from build123d import *

# Parameters (mm, degrees)
F1_DEPTH = 10.5
F3_DEPTH = 2.25
F4_R     = 1


with BuildPart() as f1:
    # F0 (on Top) → F1 (new body)
    with BuildSketch(Plane.XY):
        with BuildLine():
            Line((16, 19), (-16, 19))
            ThreePointArc((-16, 19), (-21.6568542495, 16.6568542495), (-24, 11))
            Line((-24, 11), (-24, -11))
            ThreePointArc((-24, -11), (-21.6568542495, -16.6568542495), (-16, -19))
            Line((-16, -19), (16, -19))
            ThreePointArc((16, -19), (21.6568542495, -16.6568542495), (24, -11))
            Line((24, -11), (24, 11))
            ThreePointArc((24, 11), (21.6568542495, 16.6568542495), (16, 19))
        make_face()
    extrude(amount=F1_DEPTH)

    # F2 (on face) → F3 (join)
    with BuildSketch(Plane.XY.offset(10.5)):
        with BuildLine():
            Line((10, 21.85), (-16, 21.85))
            ThreePointArc((-16, 21.85), (-21.6568542495, 19.5068542495), (-24, 13.85))
            Line((-24, 13.85), (-24, 11))
            ThreePointArc((-24, 11), (-21.6568542495, 16.6568542495), (-16, 19))
            Line((-16, 19), (10, 19))
            Line((10, 19), (10, 21.85))
        make_face()
        with BuildLine():
            Line((10, -21.85), (10, -19))
            Line((10, -19), (-16, -19))
            ThreePointArc((-16, -19), (-21.6568542495, -16.6568542495), (-24, -11))
            Line((-24, -11), (-24, -13.85))
            ThreePointArc((-24, -13.85), (-21.6568542495, -19.5068542495), (-16, -21.85))
            Line((-16, -21.85), (10, -21.85))
        make_face()
    extrude(amount=-F3_DEPTH)

    # F4
    f4_edges = [f1.edges().sort_by_distance(p)[0] for p in [
        (10, -19, 9.375),
        (10, -21.85, 9.375),
        (10, 21.85, 9.375),
        (10, 19, 9.375),
    ]]
    fillet(f4_edges, radius=F4_R)


solid = f1.part
Design review of the part built by this model. Coordinates are the model's own, in mm. A direction names the side the tool comes from. Round coordinates to 2 decimals unless told otherwise and drop trailing zeros. Loops run counter-clockwise (first coordinate to the right, second up) from the corner with the lowest first, then second, coordinate; pieces in that order, holes last. Notation, with made-up numbers: (22, 68) -> (78, 68) arc R27 cw to (78, 104) -> close; hole circle Ø11 at (63.5, -20). An arc over 180 degrees is marked (long way). Use one line per item in the form item = value. Start each with the question number.
Q1. Machinability: for faces 1 (the face through (21.594, -16.719, 5.176)), 2 (the face through (-7, -20, 8.25)), 3 (the face through (-21.594, 16.719, 4.067)), which of the approach directions +Z, -Z, +X, -X, +Y, -Y give a long, thin tool a straight path to every point of the face, cutting with its end or side? Answer none if there is none.
Q2. Wall thickness on line 1 along Y through (x, z) = (-8, 3.75); line 2 along X through (y, z) = (12, 3.25); line 3 along X through (y, z) = (16, 4) (3 decimals): over which ranges is each line inside the solid? List them lowest first. Write a range as [from, to].
Q3. We need section A-A on z = 1. Give the boundary of the cut face in (x, y), then the cut area to 3 significant figures.
Q4. We need section B-B on x = -19. Give the boundary of the cut face in (y, z).
Q5. We need section D-D on x = 18. Give the boundary of the cut face in (y, z).
Q6. For pin 1 Ø1.5 at (x, y) = (14, 6.5) entering from -Z; pin 2 Ø3 at (y, z) = (-16, 5.5) entering from +X; pin 3 Ø5 at (x, z) = (-7.5, 3.5) entering from -Y; pin 4 Ø0.7 at (y, z) = (20.5, 9) entering from +X, all flat-tipped, find the tip position at first contact; note any pin that passes through.
Q7. We need section C-C on y = -16. Give the boundary of the cut face in (x, z) (3 decimals).
Calculated:
q1.face_1 = +Z, -Z, +X, -Y
q1.face_2 = -Z, -X, -Y
q1.face_3 = -Z, -X, +Y
q2.line_1 = [-19, 19]
q2.line_2 = [-23.94, 23.94]
q2.line_3 = [-22.245, 22.245]
q3.outline = (-24, -11) arc R8 ccw to (-16, -19) -> (16, -19) arc R8 ccw to (24, -11) -> (24, 11) arc R8 ccw to (16, 19) -> (-16, 19) arc R8 ccw to (-24, 11) -> close
q3.area = 1,770 mm²
q4.outline = (-21.27, 8.25) -> (-18.42, 8.25) -> (-18.42, 0) -> (18.42, 0) -> (18.42, 8.25) -> (21.27, 8.25) -> (21.27, 10.5) -> (-21.27, 10.5) -> close
q5.outline = (-18.75, 0) -> (18.75, 0) -> (18.75, 10.5) -> (-18.75, 10.5) -> close
q6.pin_1 = 0
q6.pin_2 = 23.19
q6.pin_3 = -19
q6.pin_4 = 10
q7.outline = (-23.706, 8.25) -> (-22.245, 8.25) -> (-22.245, 0) -> (22.245, 0) -> (22.245, 10.5) -> (-23.706, 10.5) -> close
